Geometry: final body of the model. Coordinates: model frame, mm. A direction names the side the tool comes from. Round coordinates to 2 decimals unless told otherwise and drop trailing zeros. Write each loop counter-clockwise with the first axis right and the second up, starting at its lowest first coordinate (ties: lowest second). Pieces come first, ordered by that corner, then holes. Notation, with made-up numbers: M 79,72.5 L 97,72.5 A8 ccw 97,81.5 Z; hole C 60.25,17 d10. An arc over 180 degrees is marked long. Answer as CSV lines item,"result". Start each with the question number.
Q1. Reachability of faces 4 (the cylindrical face through (-9.76, 31, 64.9)), 5 (the flat face through (-47, -74, 44)), 6 (the cylindrical face through (-34, -73, 43)), 7 (the cylindrical face through (34, -73, 43)), 8 (the cylindrical face through (67.425, 35.069, 168.28)) from +Z, -Z, +X, -X, +Y, -Y: full face, straight path, thin tool, end or side. Return the list, or none.
Q2. Mould query, pull axis X, two halves, no side actions, for faces 1 (the cylindrical face through (58.034, -58.681, 164.54)), 2 (the flat face through (-1, 110, 165)), 3 (the flat face through (-32, -41, 31)). Classes: pulls with the +X half, pulls with the -X half, needs draft (parallel to the pull), parting line crosses it, or undercut.
Q3. Ray query, probe 1 along Z at (x, y) = (-56, -81); probe 2 along X at (y, z) = (0, 18); probe 3 along Y at (x, z) = (14.5, 110.5). Return the intervals inside material, ascending.
Q4. Section query A-A on z = 114. Output: boundary loops of the cut face in (x, y), and give its area (3 significant figures).
Q5. Section query D-D on x = 14. Give the number of separate pieces and of enclosed holes in the cut face, and give its area (3 significant figures).
Q6. Section query C-C on z = 144.5. Output: boundary loops of the cut face in (x, y), and give its area (3 significant figures).
Q7. Section query B-B on y = 0. Output: boundary loops of the cut face in (x, z), and give its area (3 significant figures).
Q8. First-contact query: pin 1 (25 mm diameter, centred on x = 0, y = 0, fed in from +Z); pin 2 (19.5 mm diameter, centred on x = -24, z = 128.5, fed in from +Y); pin 3 (8 mm diameter, centred on x = 41.5, y = 65, fed in from -Z); pin 4 (15.5 mm diameter, centred on x = 60.5, y = -63, fed in from -Z). Flat tips, straight axial feed; report the tip coordinate or a pass-through.
```python
from build123d import *

# Parameters (mm, degrees)
SKETCH2_W               = 140
SKETCH2_H               = 146
BOSS_EXTRUDE1_DEPTH     = 10
RIB1_REACH              = 212.656
SKETCH3_WALL_W          = 466.812236738
SKETCH3_WALL_H          = 10
BOSS_EXTRUDE2_DEPTH     = 10
BOSS_EXTRUDE3_REACH     = 276.583
SKETCH5_W               = 118
SKETCH5_H               = 13.111760598
BOSS_EXTRUDE4_DEPTH     = 5
SKETCH7_R               = 6
CUT_EXTRUDE1_DEPTH      = 265.085213911
SKETCH8_R               = 8
BOSS_EXTRUDE5_DEPTH     = 13.111760598
CUT_EXTRUDE2_REACH      = 223.54
SKETCH9_R               = 3.5
SKETCH10_R              = 15
CUT_EXTRUDE3_DEPTH      = 224.528522172
CUT_EXTRUDE4_REACH      = 223.54
CUT_EXTRUDE4_END_RADIUS = 32.5
SKETCH11_R              = 6
FILLET3_R               = 10
FILLET4_R               = 5
FILLET5_R               = 10


with BuildPart() as part:
    # Sketch1 → Revolve1 (revolve)
    with BuildSketch(Plane(origin=(0, 0, 0), x_dir=(0, 0, -1), z_dir=(1, 0, 0))):
        Polygon((0, 32.5), (-128, 32.5), (-158.888239402, 86), (-172, 86), (-172, 76), (-164.661742094, 76), (-139.547005384, 32.5), (-148, 32.5), (-148, 17.5), (-100, 17.5), (-100, 21), (-50, 21), (-50, 17.5), (0, 17.5), align=None)
    revolve(axis=Axis((0, 0, 0), (0, 0, 1)))

    # Sketch2 → Boss-Extrude1 (add)
    with BuildSketch(Plane(origin=(0, -86, 0), x_dir=(1, 0, 0), z_dir=(0, 1, 0))):
        with Locations((0, -99)):
            Rectangle(SKETCH2_W, SKETCH2_H)
    extrude(amount=BOSS_EXTRUDE1_DEPTH)

    # Sketch3 wall → Rib1 (add, up to next)
    with BuildSketch(Plane(origin=(0, -54.25, 26), x_dir=(0, 1, 0), z_dir=(0, 0, 1)), mode=Mode.PRIVATE) as rib1_sk1:
        Rectangle(SKETCH3_WALL_W, SKETCH3_WALL_H)
    rib1_tool1 = extrude(rib1_sk1.sketch, amount=RIB1_REACH, mode=Mode.PRIVATE) - part.part
    add(rib1_tool1.solids().sort_by_distance((0, -54.25, 26))[0])

    # Sketch4 → Boss-Extrude2 (add)
    with BuildSketch(Plane(origin=(0, 0, 26), x_dir=(-1, 0, 0), z_dir=(0, 0, -1))):
        with BuildLine():
            Line((-32, -76), (-32, -5.678908346))
            ThreePointArc((-32, -5.678908346), (-22.736344844, -23.223019251), (-5, -32.113081447))
            ThreePointArc((-5, -32.113081447), (0, -32.5), (5, -32.113081447))
            ThreePointArc((5, -32.113081447), (22.736344844, -23.223019251), (32, -5.678908346))
            Line((32, -5.678908346), (32, -76))
            Line((32, -76), (-32, -76))
        make_face()
    extrude(amount=-BOSS_EXTRUDE2_DEPTH)

    # Sketch5 → Boss-Extrude3 (add, up to next)
    with BuildSketch(Plane(origin=(0, 110, 0), x_dir=(1, 0, 0), z_dir=(0, 1, 0)), mode=Mode.PRIVATE) as boss_extrude3_sk1:
        with Locations((0, -165.444119701)):
            Rectangle(SKETCH5_W, SKETCH5_H)
    boss_extrude3_tool1 = extrude(boss_extrude3_sk1.sketch, amount=-BOSS_EXTRUDE3_REACH, mode=Mode.PRIVATE) - part.part
    add(boss_extrude3_tool1.solids().sort_by_distance((0, 110, 165.44412))[0])

    # Sketch6 → Boss-Extrude4 (add)
    with BuildSketch(Plane(origin=(0, -76, 0), x_dir=(1, 0, 0), z_dir=(0, 1, 0))):
        with BuildLine():
            Line((5, -36), (5, -72))
            Line((5, -72), (56, -72))
            ThreePointArc((56, -72), (70, -58), (56, -44))
            Line((56, -44), (32, -44))
            Line((32, -44), (32, -36))
            Line((32, -36), (5, -36))
        make_face()
    boss_extrude4 = extrude(amount=BOSS_EXTRUDE4_DEPTH)

    # Sketch7 → Cut-Extrude1 (cut, through all)
    with BuildSketch(Plane(origin=(0, -71, 0), x_dir=(1, 0, 0), z_dir=(0, 1, 0))):
        with Locations(Location((56, -58, 0), (0, 0, 270))):
            Circle(SKETCH7_R)
    cut_extrude1 = extrude(amount=-CUT_EXTRUDE1_DEPTH, mode=Mode.SUBTRACT)

    # Mirror1: Boss-Extrude4, Cut-Extrude1 across plane
    add(boss_extrude4.mirror(Plane(origin=(0, 0, 0), x_dir=(0, 0, 1), z_dir=(1, 0, 0))))
    add(cut_extrude1.mirror(Plane(origin=(0, 0, 0), x_dir=(0, 0, 1), z_dir=(1, 0, 0))), mode=Mode.SUBTRACT)

    # Sketch8 → Boss-Extrude5 (add)
    with BuildSketch(Plane.XY.offset(172)):
        with Locations((-60.811183182, 60.811183182)):
            Circle(SKETCH8_R)
        with Locations((60.811183182, 60.811183182)):
            Circle(SKETCH8_R)
    boss_extrude5 = extrude(amount=-BOSS_EXTRUDE5_DEPTH)

    # Sketch9 → Cut-Extrude2 (cut, up to next)
    with BuildSketch(Plane.XY.offset(172), mode=Mode.PRIVATE) as cut_extrude2_sk1:
        with Locations((-60.811183182, 60.811183182)):
            Circle(SKETCH9_R)
    cut_extrude2_tool1 = extrude(cut_extrude2_sk1.sketch, amount=-CUT_EXTRUDE2_REACH, mode=Mode.PRIVATE) & part.part
    # Sketch9 → Cut-Extrude2 (cut, up to next)
    with BuildSketch(Plane.XY.offset(172), mode=Mode.PRIVATE) as cut_extrude2_sk2:
        with Locations((60.811183182, 60.811183182)):
            Circle(SKETCH9_R)
    cut_extrude2_tool2 = extrude(cut_extrude2_sk2.sketch, amount=-CUT_EXTRUDE2_REACH, mode=Mode.PRIVATE) & part.part
    cut_extrude2_1 = cut_extrude2_tool1.solids().sort_by_distance((-60.811183, 60.811183, 172))[0]
    add(cut_extrude2_1, mode=Mode.SUBTRACT)
    cut_extrude2_2 = cut_extrude2_tool2.solids().sort_by_distance((60.811183, 60.811183, 172))[0]
    add(cut_extrude2_2, mode=Mode.SUBTRACT)
    cut_extrude2 = cut_extrude2_1 + cut_extrude2_2  # Cut-Extrude2 as one shape, for the pattern or mirror that repeats it

    # Mirror2: Boss-Extrude5, Cut-Extrude2 across plane
    add(boss_extrude5.mirror(Plane.ZX))
    add(cut_extrude2.mirror(Plane.ZX), mode=Mode.SUBTRACT)

    # Sketch10 → Cut-Extrude3 (cut, through all)
    with BuildSketch(Plane(origin=(5, 0, 0), x_dir=(0, 0, -1), z_dir=(1, 0, 0))):
        with Locations((-114, -56)):
            Circle(SKETCH10_R)
    extrude(amount=-CUT_EXTRUDE3_DEPTH, mode=Mode.SUBTRACT)

    # Cut-Extrude4: up to this cylinder (the profile starts inside it)
    cut_extrude4_end = Plane(origin=(0, 0, 36), z_dir=(0, 0, -1)) * Cylinder(CUT_EXTRUDE4_END_RADIUS, 513.08, mode=Mode.PRIVATE)
    # Sketch11 → Cut-Extrude4 (cut, up to the surface)
    with BuildSketch(Plane(origin=(0, 0, 0), x_dir=(1, 0, 0), z_dir=(0, 1, 0)), mode=Mode.PRIVATE) as cut_extrude4_sk1:
        with Locations(Location((0, -36, 0), (0, 0, 90))):
            Circle(SKETCH11_R)
    cut_extrude4_tool1 = extrude(cut_extrude4_sk1.sketch, amount=CUT_EXTRUDE4_REACH, mode=Mode.PRIVATE) & cut_extrude4_end
    add(cut_extrude4_tool1.solids().sort_by_distance((0, 0, 36))[0], mode=Mode.SUBTRACT)

    # Fillet3
    fillet3_edges = [part.edges().sort_by_distance(p)[0] for p in [
        (-59, 110, 165.444119701),
        (59, 110, 165.444119701),
    ]]
    fillet(fillet3_edges, radius=FILLET3_R)

    # Fillet4
    fillet4_edges = [part.edges().sort_by_distance(p)[0] for p in [
        (32, -73.5, 44),
        (5, -73.5, 72),
        (-5, -73.5, 72),
        (-32, -73.5, 44),
    ]]
    fillet(fillet4_edges, radius=FILLET4_R)

    # Fillet5
    fillet5_edges = [part.edges().sort_by_distance(p)[0] for p in [
        (-70, -81, 172),
        (-70, -81, 26),
        (70, -81, 172),
        (70, -81, 26),
    ]]
    fillet(fillet5_edges, radius=FILLET5_R)


solid = part.part
```
Entries:
1,face 4,"none"
1,face 5,"-Z, -X, +Y"
1,face 6,"-Z, -X"
1,face 7,"-Z, +X"
1,face 8,"+Z"
2,face 1,"undercut"
2,face 2,"needs draft"
2,face 3,"pulls with the -X half"
3,probe 1,"z = 26 to 52, 64 to 172"
3,probe 2,"x = -32.5 to -17.5, 17.5 to 32.5"
3,probe 3,"y = -86 to -76, -29.09 to -9.8, 9.8 to 29.09"
4,outline,"M -70,-86 L 70,-86 L 70,-76 L 5,-76 L 5,-71 L -5,-71 L -5,-76 L -70,-76 Z; M -5,-41 L 5,-41 L 5,-32.11 A32.5 ccw long -5,-32.11 Z; hole C 0,0 d35"
4,area,"3,890 mm^2"
5,separate pieces,"2"
5,enclosed holes,"1"
5,area,"8,730 mm^2"
6,outline,"M -70,-86 L 70,-86 L 70,-76 L 5,-76 L 5,-60.87 A61.08 ccw long -5,-60.87 L -5,-76 L -70,-76 Z; C 0,0 d65; hole C 0,0 d82.16; hole C 0,0 d35"
6,area,"10,300 mm^2"
7,outline,"M -86,158.89 L -32.5,128 L -32.5,0 L -17.5,0 L -17.5,50 L -21,50 L -21,100 L -17.5,100 L -17.5,148 L -32.5,148 L -32.5,139.55 L -76,164.66 L -76,172 L -86,172 Z; M 17.5,0 L 32.5,0 L 32.5,128 L 86,158.89 L 86,172 L 76,172 L 76,164.66 L 32.5,139.55 L 32.5,148 L 17.5,148 L 17.5,100 L 21,100 L 21,50 L 17.5,50 Z"
7,area,"5,410 mm^2"
8,pin 1,"passes through"
8,pin 2,"stops at y = 44.8"
8,pin 3,"stops at z = 151.45"
8,pin 4,"stops at z = 155.19"
